Could you check a few things on this model? Use its own coordinates, in mm. A direction names the side the tool comes from. Give positions to 0.01 mm unless a question says otherwise; leave off trailing zeros. Loops run counter-clockwise (first coordinate to the right, second up) from the corner with the lowest first, then second, coordinate; pieces in that order, holes last. Notation, with made-up numbers: (-33, -39.5) -> (-27, -39.5) arc R30 ccw to (-27, -4.5) -> close; hole circle Ø9 at (33.25, -2). An arc over 180 degrees is marked (long way). Write item = value, one per line. Start each with the question number.
1) I want a section at B-B (y = -5.25). List the corners of the cut face in (x, z) for me, and give its area (3 significant figures).
2) I want a section at D-D (x = -11.5). List the corners of the cut face in (y, z) for me, and give its area (3 significant figures).
3) I need wall thicknesses on probe 1 along X at (y, z) = (5, 2.75); probe 2 along Y at (x, z) = (-4.25, 4.5); probe 3 along Y at (x, z) = (7.5, 1.5) (3 decimals). Which ranges of each line are inside material? Lowest first, please. Write a range as from..to.
4) I want a section at A-A (x = 7.5). List the corners of the cut face in (y, z) for me (3 decimals).
5) On a 3-axis mill with a long thin cutter (end or side, diameter ignored), from which of +Z, -Z, +X, -X, +Y, -Y can I reach the whole of each face in a straight line? I mean faces 3 (the face through (-8.261, 4.188, 3.204)), 4 (the face through (-12, 0, 3)). Say none if no direction works.
6) I'm going to push a flat-ended pin straight in: pin 1 Ø4 at (x, y) = (4.7, -0.025) entering from -Z. Where does the tip first touch, or does it pass through?
7) If we mould it in two halves opening along Y, with no side actions, what happens to faces 1 (the face through (0, 7, 0)), 2 (the face through (7.72, 4.1, 3.2))? For each: +Y half, -Y half, draft (parallel to the pull), parting line (faces both ways), or undercut.
8) I want a section at C-C (y = 1). List the corners of the cut face in (x, z) for me.
from build123d import *

# Parameters (mm, degrees)
ESBO_O1_W                = 28
ESBO_O1_H                = 15
RESSALTO_EXTRUS_O1_DEPTH = 6.5
ESBO_O2_W                = 20
ESBO_O2_H                = 5.5
CORTE_EXTRUS_O1_DEPTH    = 5.5
ESBO_O3_R                = 1
CORTE_EXTRUS_O2_DEPTH    = 18.161002302
CORTE_EXTRUS_O3_DEPTH    = 5.5
CORTE_EXTRUS_O4_DEPTH    = 5.5
ESBO_O6_W                = 2
ESBO_O6_H                = 5.5
CORTE_EXTRUS_O5_DEPTH    = 5.5
ESBO_O7_R                = 1.5
CORTE_EXTRUS_O6_DEPTH    = 5.5
FILETE1_R                = 0.5
FILETE2_R                = 0.5


with BuildPart() as part:
    # Esboço1 → Ressalto-extrusão1 (new body)
    with BuildSketch(Plane.XY):
        Rectangle(ESBO_O1_W, ESBO_O1_H)
    extrude(amount=RESSALTO_EXTRUS_O1_DEPTH)

    # Esboço2 → Corte-extrusão1 (cut)
    with BuildSketch(Plane(origin=(0, 0, 0), x_dir=(-1, 0, 0), z_dir=(0, 0, -1))):
        Rectangle(ESBO_O2_W, ESBO_O2_H)
    extrude(amount=-CORTE_EXTRUS_O1_DEPTH, mode=Mode.SUBTRACT)

    # Esboço3 → Corte-extrusão2 (cut, through all)
    with BuildSketch(Plane(origin=(0, 0, 0), x_dir=(-1, 0, 0), z_dir=(0, 0, -1))):
        with Locations((-7.5, 5.075)):
            Circle(ESBO_O3_R)
        with Locations((7.8, 5.075)):
            Circle(ESBO_O3_R)
        with Locations((-12.1, -3.125)):
            Circle(ESBO_O3_R)
    extrude(amount=-CORTE_EXTRUS_O2_DEPTH, mode=Mode.SUBTRACT)

    # Esboço4 → Corte-extrusão3 (cut)
    with BuildSketch(Plane(origin=(0, 0, 0), x_dir=(-1, 0, 0), z_dir=(0, 0, -1))):
        Polygon((0, -2.75), (-5, -2.75), (-5, -6), (5, -6), (5, -2.75), align=None)
    extrude(amount=-CORTE_EXTRUS_O3_DEPTH, mode=Mode.SUBTRACT)

    # Esboço5 → Corte-extrusão4 (cut)
    with BuildSketch(Plane(origin=(0, 0, 0), x_dir=(-1, 0, 0), z_dir=(0, 0, -1))):
        Polygon((0, 2.75), (-5, 2.75), (-5, 6), (5, 6), (5, 2.75), align=None)
    extrude(amount=-CORTE_EXTRUS_O4_DEPTH, mode=Mode.SUBTRACT)

    # Esboço6 → Corte-extrusão5 (cut)
    with BuildSketch(Plane(origin=(0, 0, 0), x_dir=(-1, 0, 0), z_dir=(0, 0, -1))):
        with Locations((11, 0)):
            Rectangle(ESBO_O6_W, ESBO_O6_H)
    extrude(amount=-CORTE_EXTRUS_O5_DEPTH, mode=Mode.SUBTRACT)

    # Esboço7 → Corte-extrusão6 (cut)
    with BuildSketch(Plane.XY.offset(6.5)):
        with Locations((-5, 0)):
            Circle(ESBO_O7_R)
        with Locations((4.7, -0.025)):
            Circle(ESBO_O7_R)
    extrude(amount=-CORTE_EXTRUS_O6_DEPTH, mode=Mode.SUBTRACT)

    # Filete1
    filete1_edges = [part.edges().sort_by_distance(p)[0] for p in [
        (-14, 0, 6.5),
        (0, -7.5, 6.5),
        (14, 0, 6.5),
        (0, 7.5, 6.5),
    ]]
    fillet(filete1_edges, radius=FILETE1_R)

    # Filete2
    filete2_edges = [part.edges().sort_by_distance(p)[0] for p in [
        (10, 0, 0),
        (7.5, -2.75, 0),
        (-8.5, 2.75, 0),
        (-8.5, -2.75, 0),
        (-5, -4.375, 0),
        (5, -4.375, 0),
        (0, -6, 0),
        (7.5, 2.75, 0),
        (-5, 4.375, 0),
        (0, 6, 0),
        (5, 4.375, 0),
        (-12, 0, 0),
    ]]
    fillet(filete2_edges, radius=FILETE2_R)


solid = part.part
Answer list:
q1.outline = (-14, 0) -> (-5.5, 0) arc R0.5 ccw to (-5, 0.5) -> (-5, 5.5) -> (5, 5.5) -> (5, 0.5) arc R0.5 ccw to (5.5, 0) -> (14, 0) -> (14, 6) arc R0.5 ccw to (13.5, 6.5) -> (-13.5, 6.5) arc R0.5 ccw to (-14, 6) -> close
q1.area = 127 mm^2
q2.outline = (-7.5, 0) -> (-3.25, 0) arc R0.5 ccw to (-2.75, 0.5) -> (-2.75, 5.5) -> (2.75, 5.5) -> (2.75, 0.5) arc R0.5 ccw to (3.25, 0) -> (7.5, 0) -> (7.5, 6) arc R0.5 ccw to (7, 6.5) -> (-7, 6.5) arc R0.5 ccw to (-7.5, 6) -> close
q2.area = 67.0 mm^2
q3.probe_1 = -14..-8.8, -6.8..-5, 5..6.5, 8.5..14
q3.probe_2 = -7.5..-6, 6..7.5
q3.probe_3 = -7.5..-2.75, 2.75..4.075, 6.075..7.5
q4.outline = (-7.5, 0) -> (-3.25, 0) arc R0.5 ccw to (-2.75, 0.5) -> (-2.75, 5.5) -> (2.75, 5.5) -> (2.75, 0.5) arc R0.5 ccw to (3.25, 0) -> (4.075, 0) -> (4.075, 6.5) -> (-7, 6.5) arc R0.5 ccw to (-7.5, 6) -> close; (6.075, 0) -> (7.5, 0) -> (7.5, 6) arc R0.5 ccw to (7, 6.5) -> (6.075, 6.5) -> close
q5.face_3 = +Z, -Z
q5.face_4 = -Z
q6.pin_1 = 5.5
q7.face_1 = draft
q7.face_2 = undercut
q8.outline = (-14, 0) -> (-12.5, 0) arc R0.5 ccw to (-12, 0.5) -> (-12, 5.5) -> (-6.12, 5.5) -> (-6.12, 6.5) -> (-13.5, 6.5) arc R0.5 ccw to (-14, 6) -> close; (-3.88, 5.5) -> (3.6, 5.5) -> (3.6, 6.5) -> (-3.88, 6.5) -> close; (5.8, 5.5) -> (10, 5.5) -> (10, 0.5) arc R0.5 ccw to (10.5, 0) -> (14, 0) -> (14, 6) arc R0.5 ccw to (13.5, 6.5) -> (5.8, 6.5) -> close
